Autodesk Inventor part; units mm, degrees
ref_plane "YZ Plane" through (0, 0, 0) normal (1, 0, 0) x (0, 1, 0)
ref_plane "XZ Plane" through (0, 0, 0) normal (0, 1, 0) x (-1, 0, 0)
ref_plane "XY Plane" through (0, 0, 0) normal (0, 0, 1) x (1, 0, 0)
sketch "Sketch1" plane through (0, 0, 0) normal (0, 0, 1) x (1, 0, 0)
  circle A0 centre (0, 0) radius 292.1
  line L0 (-292.1, 0) -> (-266.7, 0)
  line L1 (-292.1, 0) -> (-317.5, 0)
  circle A1 centre (0, 0) radius 317.5
  line L2 (-317.5, 0) -> (-317.5, -127)
  line L3 (-317.5, -127) -> (-263.0464, -127)
  circle A2 centre (0, 0) radius 317.5
  dimension "d0" = 584.2
  dimension "d1" = 25.4
  dimension "d2" = 25.4
  dimension "d3" = 127
extrude "Extrusion1" add sketch "Sketch1" along normal blind 12.7 contours A0 L3 A1 L1 | A1 L3 L2 picked at (-275.2864, -120.3141)
sketch "Sketch2" plane through (0, 0, 12.7) normal (0, 0, 1) x (1, 0, 0)
  line L0 (-317.5, 0) -> (-317.5, -127)
  line L1 (-317.5, -127) -> (-263.0464, -127)
  arc A0 (-292.1, 0) -> (-263.0464, -127) centre (0, 0) ccw
  circle A1 centre (0, 0) radius 292.1
  circle A2 centre (0, 0) radius 317.5
  line L2 (-317.5, 0) -> (-317.5, -127)
  line L3 (-317.5, -127) -> (-290.9936, -127)
extrude "Extrusion2" cut sketch "Sketch2" against normal blind 25.4 contours A2 L1 L0
sketch "Sketch3" plane through (0, 0, 12.7) normal (0, 0, 1) x (1, 0, 0)
  arc A0 (-317.5, 0) -> (-290.9936, -127) centre (0, 0) ccw
  line L0 (-290.9936, -127) -> (-316.1859, -127)
  line L1 (-295.9122, -115.0749) -> (-295.9122, -127)
  line L2 (-281.9422, -117.475) -> (-276.8622, -117.475)
  line L3 (-276.8622, -117.475) -> (-276.8622, -123.825)
  line L4 (-276.8622, -123.825) -> (-287.0222, -123.825)
  line L5 (-287.0222, -123.825) -> (-287.0222, -117.475)
  line L6 (-287.0222, -117.475) -> (-281.9422, -117.475)
  line L7 (-290.9936, -127) -> (-263.0464, -127)
  dimension "d16" = 5.08
  dimension "d17" = 6.35
  dimension "d18" = 10.16
  dimension "d20" = 4.9186
  dimension "d33" = 13.97
  dimension "d34" = 9.525
  dimension "d35" = 8.89
extrude "Extrusion3" cut sketch "Sketch3" against normal blind 25.4
sketch "Sketch4" plane through (0, 0, 12.7) normal (0, 0, 1) x (1, 0, 0)
  arc A0 (-317.5, 0) -> (-290.9936, -127) centre (0, 0) ccw
  arc A1 (-292.1, 0) -> (-263.0464, -127) centre (0, 0) ccw
  line L0 (-292.1, 0) -> (-317.5, 0)
  line L1 (-317.5, 0) -> (-317.5, 25.4)
  line L2 (-317.5, 25.4) -> (-292.1, 25.4)
  line L3 (-292.1, 25.4) -> (-292.1, 0)
  line L4 (-317.5, 0) -> (-292.1, 0)
  dimension "d24" = 25.4
extrude "Extrusion4" add sketch "Sketch4" against normal blind 12.7
sketch "Sketch5" plane through (0, 0, 12.7) normal (0, 0, 1) x (1, 0, 0)
  line L0 (-292.1, 0) -> (-292.1, 25.4)
  line L1 (-292.1, 25.4) -> (-317.5, 25.4)
  line L2 (-317.5, 25.4) -> (-317.5, 0)
  line L3 (-304.8, 25.4) -> (-304.8, 22.225)
  line L4 (-304.8, 22.225) -> (-299.72, 22.225)
  line L5 (-299.72, 22.225) -> (-299.72, 15.875)
  line L6 (-299.72, 15.875) -> (-309.88, 15.875)
  line L7 (-309.88, 15.875) -> (-309.88, 22.225)
  line L8 (-309.88, 22.225) -> (-304.8, 22.225)
  dimension "d27" = 3.175
  dimension "d28" = 5.08
  dimension "d29" = 6.35
  dimension "d30" = 10.16
extrude "Extrusion5" cut sketch "Sketch5" against normal blind 254
sketch "Sketch6" plane through (0, 0, 12.7) normal (0, 0, 1) x (1, 0, 0)
  line L0 (-290.9936, -127) -> (-263.0464, -127)
  arc A0 (-292.1, 0) -> (-263.0464, -127) centre (0, 0) ccw
  line L1 (-290.9936, -127) -> (-270.6736, -127)
  line L2 (-270.6736, -127) -> (-270.6736, -109.81)
  line L3 (-270.6736, -109.81) -> (-256.8603, -109.81)
  line L4 (-256.8603, -109.81) -> (-256.8603, -127)
  line L5 (-256.8603, -127) -> (-270.6736, -127)
  dimension "d36" = 20.32
  dimension "d37" = 13.8133
extrude "Extrusion6" cut sketch "Sketch6" against normal blind 254 contours L2 A0 L0
sketch "Sketch7" plane through (0, 0, 12.7) normal (0, 0, 1) x (1, 0, 0)
  arc A0 (-317.5, 0) -> (-290.9936, -127) centre (0, 0) ccw
  line L0 (-276.8622, -117.475) -> (-276.8622, -123.825)
  line L1 (-317.5, 0) -> (-317.5, -127) construction
  line L2 (-317.5, -63.5) -> (-317.5, -50.8) construction
  line L3 (-317.5, -50.8) -> (-317.5, -38.1) construction
  line L4 (-317.5, -38.1) -> (-317.5, -25.4) construction
  line L5 (-317.5, -25.4) -> (-317.5, -12.7) construction
  line L6 (-317.5, 23.7649) -> (-317.5, -16.9672) construction
  line L7 (-317.5, -16.9672) -> (-180.5967, -16.9672) construction
  line L8 (-317.5, -16.9672) -> (-309.2958, -16.9672) construction
  line L9 (-309.2958, -16.9672) -> (-309.2958, -23.3172)
  line L10 (-309.2958, -23.3172) -> (-299.1358, -23.3172)
  line L11 (-299.1358, -23.3172) -> (-299.1358, -16.9672)
  line L12 (-309.2958, -16.9672) -> (-299.1358, -16.9672)
  point P0 (-317.5, 25.4)
  dimension "d59" = 8.2042
  dimension "d60" = 6.35
  dimension "d61" = 10.16
  dimension "d65" = 42.3672
extrude "Extrusion8" cut sketch "Sketch7" against normal blind 25.4
properties part number "HopperFrontSupport_v2"
Verification items for the finished model (mm, model axes). A direction names the side the tool comes from. Coordinates: 2 decimals unless noted, no trailing zeros. Loops run counter-clockwise (first coordinate to the right, second up) from the corner with the lowest first, then second, coordinate; pieces in that order, holes last. Notation, with made-up numbers: (65, -27) -> (87, -27) arc R25 cw to (87, -4) -> close; hole circle Ø5 at (2.5, 12). An arc over 180 degrees is marked (long way). Answer in a Markdown table with one row per item. Add a question column.
1. Section check A-A, the plane z = 5.5. Enter the section's corners in (x, y) (3 decimals).
2. Section check D-D, the plane y = 10. Enter the section's corners in (x, z), then the cut area to 3 significant figures.
3. Section check C-C, the plane x = -283.5. Enter the section's corners in (y, z) (3 decimals).
4. Material ranges on probe 1 along X at (y, z) = (16, 1.5); probe 2 along X at (y, z) = (-119, 4.25); probe 3 along Y at (x, z) = (-292.5, 4), recorded low to high. Write a range as [from, to].
5. Section check B-B, the plane x = -306. Enter the section's corners in (y, z) (3 decimals), then the cut area to 3 significant figures.
6. Draft check along X on faces 1 (the face through (-287.022, -121, 6)), 2 (the face through (-305, 25.4, 6)), 3 (the face through (-317.5, 13, 6)). Enter one of: +X half, -X half, draft (parallel to the pull), parting line (faces both ways), or undercut.
7. Depth check by flat-ended pin: P1, Ø1.5, axis at y = -37.5, z = 10, coming from the +X side; P2, Ø3, axis at y = -21, z = 4, coming from the +X side; P3, Ø1.9, axis at y = 17.5, z = 5.5, coming from the +X side. Enter the tip coordinate at first touch or a pass-through.
8. Access from +Z, -Z, +X, -X, +Y, -Y to the whole of each face (thin tool, end or side, straight path). Record for faces 4 (the face through (-292.1, 13, 6)), 5 (the face through (-281, -127, 6)), 6 (the face through (-282, -123.825, 6)).
Derived:
| question | item | result |
|---|---|---|
| 1 | outline | (-317.5, 0) arc R317.5 ccw to (-290.994, -127) -> (-270.674, -127) -> (-270.674, -109.81) arc R292.1 cw to (-292.1, 0) -> (-292.1, 25.4) -> (-317.5, 25.4) -> close; hole (-309.88, 15.875) -> (-299.72, 15.875) -> (-299.72, 22.225) -> (-309.88, 22.225) -> close; hole (-309.296, -23.317) -> (-299.136, -23.317) -> (-299.136, -16.967) -> (-309.296, -16.967) -> close; hole (-287.022, -123.825) -> (-276.862, -123.825) -> (-276.862, -117.475) -> (-287.022, -117.475) -> close |
| 2 | outline | (-317.5, 0) -> (-292.1, 0) -> (-292.1, 12.7) -> (-317.5, 12.7) -> close |
| 2 | area | 323 mm² |
| 3 | outline | (-127, 0) -> (-123.825, 0) -> (-123.825, 12.7) -> (-127, 12.7) -> close; (-117.475, 0) -> (-70.357, 0) -> (-70.357, 12.7) -> (-117.475, 12.7) -> close |
| 4 | probe 1 | x = [-317.5, -309.88], [-299.72, -292.1] |
| 4 | probe 2 | x = [-294.36, -287.02], [-276.86, -270.67] |
| 4 | probe 3 | y = [-123.49, 25.4] |
| 5 | outline | (-84.677, 0) -> (-23.317, 0) -> (-23.317, 12.7) -> (-84.677, 12.7) -> close; (-16.967, 0) -> (15.875, 0) -> (15.875, 12.7) -> (-16.967, 12.7) -> close; (22.225, 0) -> (25.4, 0) -> (25.4, 12.7) -> (22.225, 12.7) -> close |
| 5 | area | 1,240 mm² |
| 6 | face 1 | undercut |
| 6 | face 2 | draft |
| 6 | face 3 | -X half |
| 7 | P1 | stops at x = -289.58 |
| 7 | P2 | stops at x = -291.23 |
| 7 | P3 | stops at x = -292.1 |
| 8 | face 4 | +Z, -Z, +X, +Y |
| 8 | face 5 | +Z, -Z, +X, -X, -Y |
| 8 | face 6 | +Z, -Z |
